from build123d import *

# Parameters (mm, degrees)
SKETCH1_R           = 6.5
BOSS_EXTRUDE1_DEPTH = 6
BOSS_EXTRUDE2_DEPTH = 13
SKETCH3_R           = 1.5875
CUT_EXTRUDE1_DEPTH  = 10


with BuildPart() as part:
    # Sketch1 → Boss-Extrude1 (new body)
    with BuildSketch(Plane.XY):
        Circle(SKETCH1_R)
    extrude(amount=BOSS_EXTRUDE1_DEPTH)

    # Sketch2 → Boss-Extrude2 (add)
    with BuildSketch(Plane.XY.offset(6)):
        with BuildLine():
            Line((-2.449489743, 2.5), (2.449489743, 2.5))
            ThreePointArc((2.449489743, 2.5), (3.5, 0), (2.449489743, -2.5))
            Line((2.449489743, -2.5), (-2.449489743, -2.5))
            ThreePointArc((-2.449489743, -2.5), (-3.5, 0), (-2.449489743, 2.5))
        make_face()
    extrude(amount=BOSS_EXTRUDE2_DEPTH)

    # Sketch3 → Cut-Extrude1 (cut)
    with BuildSketch(Plane(origin=(0, 0, 0), x_dir=(-1, 0, 0), z_dir=(0, 0, -1))):
        Circle(SKETCH3_R)
    extrude(amount=-CUT_EXTRUDE1_DEPTH, mode=Mode.SUBTRACT)


solid = part.part
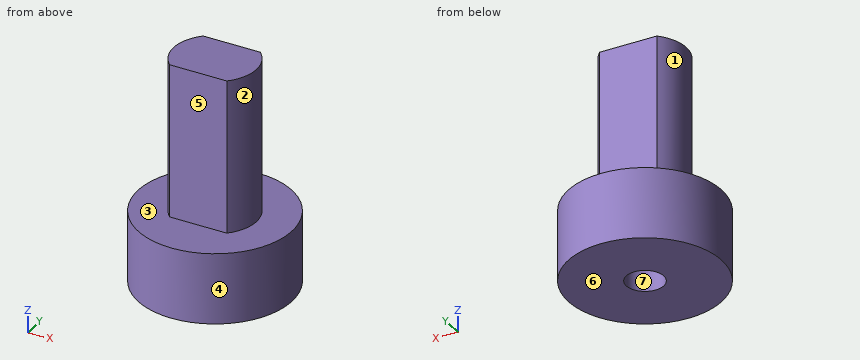
The listing builds one solid part. Answer for the finished solid, in the listing's coordinates (mm). Face numbers are marked on the shaded views. A direction names the side the tool comes from. Give positions to 0.01 mm unless a question says otherwise; leave off trailing zeros. Order: outer loops, then holes, each group sorted by start corner. A loop starts at its lowest first (then second) coordinate and runs counter-clockwise, first axis right, second up. Notation, with made-up numbers: (-7, 27) - (42, 27) arc R10 cw to (42, 33) - close; hole circle Ø1 at (-10, -32.5). An arc over 180 degrees is marked (long way). Answer as CSV lines item,"result".
Q1. A cutting plane is placed at D-D, the plane z = 11.5. Determine the outline of the cut face in (x, y).
Answer key:
outline,"(-2.45, -2.5) - (2.45, -2.5) arc R3.5 ccw to (2.45, 2.5) - (-2.45, 2.5) arc R3.5 ccw to start"
Q2. Determine the mould class of the marked faces 4, 5, 6 and 7 for opening direction Y: pulls with the +Y half, pulls with the -Y half, needs draft (parallel to the pull), parting line crosses it, or undercut.
Answer key:
face 4,"parting line crosses it"
face 5,"pulls with the -Y half"
face 6,"needs draft"
face 7,"undercut"
Q3. A cutting plane is placed at B-B, the plane y = 0. Determine the outline of the cut face in (x, z), and give its area (3 significant figures).
Answer key:
outline,"(-6.5, 0) - (-1.59, 0) - (-1.59, 10) - (1.59, 10) - (1.59, 0) - (6.5, 0) - (6.5, 6) - (3.5, 6) - (3.5, 19) - (-3.5, 19) - (-3.5, 6) - (-6.5, 6) - close"
area,"137 mm^2"
Q4. A cutting plane is placed at C-C, the plane z = 8.75. Determine the outline of the cut face in (x, y) (1 decimal).
Answer key:
outline,"(-2.4, -2.5) - (2.4, -2.5) arc R3.5 ccw to (2.4, 2.5) - (-2.4, 2.5) arc R3.5 ccw to start; hole circle Ø3.2 at (0, 0)"
Q5. Straight lines are drawn through the part: L1, parallel to Y at x = 0, z = 3.75; L2, parallel to Z at x = 0.75, y = 4.25; L3, parallel to X at y = -1.25, z = 1.5. For each, find the intervals that lie inside material, in ascending order.
Answer key:
L1,"y = -6.5 to -1.59, 1.59 to 6.5"
L2,"z = 0 to 6"
L3,"x = -6.38 to -0.98, 0.98 to 6.38"
Q6. Each of these flat-tipped pins is pushed along its axis until it touches: pin 1 Ø6 at (y, z) = (5, 6) entering from +X; pin 2 Ø5 at (x, z) = (-4.5, 7) entering from -Y; pin 3 Ø4 at (x, z) = (0.5, 10) entering from +Y; pin 4 Ø3 at (y, z) = (4.5, 13) entering from -X. Where does it stop, or does it pass through?
Answer key:
pin 1,"stops at x = 6.18"
pin 2,"stops at y = -6.11"
pin 3,"stops at y = 2.5"
pin 4,"passes through"
Q7. Which of the six approach directions +Z, -Z, +X, -X, +Y, -Y give full straight-line access (tool end or side, diameter ignored) to the marked faces 1, 2 and 3?
Answer key:
face 1,"+Z, -X"
face 2,"+Z, +X"
face 3,"+Z"
Q8. A cutting plane is placed at A-A, the plane x = 0. Determine the outline of the cut face in (y, z), and give its area (3 significant figures).
Answer key:
outline,"(-6.5, 0) - (-1.59, 0) - (-1.59, 10) - (1.59, 10) - (1.59, 0) - (6.5, 0) - (6.5, 6) - (2.5, 6) - (2.5, 19) - (-2.5, 19) - (-2.5, 6) - (-6.5, 6) - close"
area,"111 mm^2"
